Here's how the part is built. I have some questions about the finished solid (model axes, mm). A direction names the side the tool comes from. Round coordinates to 2 decimals unless told otherwise and drop trailing zeros. Loops run counter-clockwise (first coordinate to the right, second up) from the corner with the lowest first, then second, coordinate; pieces in that order, holes last. Notation, with made-up numbers: M 0.25,8 L 47.25,8 A26 ccw 47.25,32 Z; hole C 45,85 d11. An arc over 180 degrees is marked long. Write item = value, one per line. Start each with the question number.
Autodesk Inventor part; units mm, degrees
ref_plane "YZ Plane" through (0, 0, 0) normal (1, 0, 0) x (0, 1, 0)
ref_plane "XZ Plane" through (0, 0, 0) normal (0, 1, 0) x (-1, 0, 0)
ref_plane "XY Plane" through (0, 0, 0) normal (0, 0, 1) x (1, 0, 0)
sketch "Sketch1" plane through (0, 0, 0) normal (0, 0, 1) x (1, 0, 0)
  circle A0 centre (1.9343, 0.0365) radius 1.25 construction
  line L0 (0.6843, -5.4635) -> (3.1843, -5.4635)
  line L1 (3.1843, -5.4635) -> (3.1843, 5.5365)
  line L2 (3.1843, 5.5365) -> (0.6843, 5.5365)
  line L3 (0.6843, 5.5365) -> (0.6843, -5.4635)
  line L4 (0.6843, -5.4635) -> (3.1843, 5.5365) construction
  line L5 (3.1843, -5.4635) -> (0.6843, 5.5365) construction
  point P0 (0, 0)
  dimension "d0" = 11
  dimension "d1" = 2.5
extrude "Extrusion1" add sketch "Sketch1" along normal blind 2
sketch "Sketch2" plane through (3.1843, -5.4635, 0) normal (1, 0, 0) x (0, 0, -1)
  line L0 (-2, 0) -> (-2, 11)
  line L1 (-2, 0) -> (-2, 11)
  line L2 (-2, 5.5) -> (-7, 5.5)
  arc A0 (-2, 11) -> (-2, 0) centre (-1.475, 5.5) ccw
  line L3 (-2, 0) -> (-2, 1.5)
  line L4 (-2, 11) -> (-2, 9.5)
  line L5 (-7, 5.5) -> (-5.5, 5.5)
  arc A1 (-2, 9.5) -> (-2, 1.5) centre (-1.475, 5.5) ccw
  point P0 (0, 5.4635)
  dimension "d4" = 5
  dimension "d5" = 1.5
  dimension "d6" = 1.5
  dimension "d7" = 1.5
extrude "Extrusion2" add sketch "Sketch2" against normal up to surface (2.5 mm away) contours A0 L2 A1 L0 | A0 L0 A1 L2
equation "\"d6\" = d5"
equation "\"d7\" = d5"
properties part number "hook_loop"
Item 1: Will these pins go through, and if not, where does the flat tip stop? pin 1 Ø1 at (x, z) = (1.5, 3.5) entering from -Y; pin 2 Ø1.5 at (x, z) = (1, 4) entering from -Y.
Item 2: Please list where these lines run through material, in increasing order: line 1 (Z direction, x = 1.05, y = 0); line 2 (Y direction, x = 2.75, z = 2.5); line 3 (Z direction, x = 1.6, y = -3.5). Write a range as [from, to].
Item 3: For faces 1 (the flat face through (2, -5.464, 1)), 2 (the flat face through (2, 0, 2)), which set-ups out of +Z, -Z, +X, -X, +Y, -Y let a thin tool reach every point of the face, with its end or its side?
Item 4: I want a section at D-D, the plane y = -4.25. List the corners of the cut face in (x, z) for me.
Item 5: I want a section at C-C, the plane y = 0.25. List the corners of the cut face in (x, z) for me, then the cut area to 3 significant figures.
Item 6: I want a section at B-B, the plane z = 2.25. List the corners of the cut face in (x, y) for me.
Worked out:
q1.pin_1 = -5.27
q1.pin_2 = -5.2
q2.line_1 = [0, 2], [5.51, 7]
q2.line_2 = [-5.39, -3.87], [3.94, 5.47]
q2.line_3 = [0, 2], [3.42, 5.72]
q3.face_1 = +Z, -Z, +X, -X, -Y
q3.face_2 = +X, -X
q4.outline = M 0.68,0 L 3.18,0 L 3.18,4.96 L 0.68,4.96 Z
q5.outline = M 0.68,0 L 3.18,0 L 3.18,2 L 0.68,2 Z; M 0.68,5.5 L 3.18,5.5 L 3.18,7 L 0.68,7 Z
q5.area = 8.73 mm2
q6.outline = M 0.68,-5.43 L 3.18,-5.43 L 3.18,-3.92 L 0.68,-3.92 Z; M 0.68,4 L 3.18,4 L 3.18,5.51 L 0.68,5.51 Z
